The drawing under review shows one solid part. Ordinate dimensions are in mm from its lowest x, y, z. Give positions to 0.01 mm unless a question says otherwise; leave off trailing zeros. Write each loop counter-clockwise with the first axis right and the second up, starting at its lowest first coordinate (ties: lowest second). Pieces come first, ordered by that corner, then holes. Notation, with made-up numbers: M -16.75,18 L 36.25,18 A7 cw 36.25,24 Z; hole C 7,25.25 d10. An arc over 180 degrees is marked long. Answer as a JSON object with one key per item and string values. Group by question number.
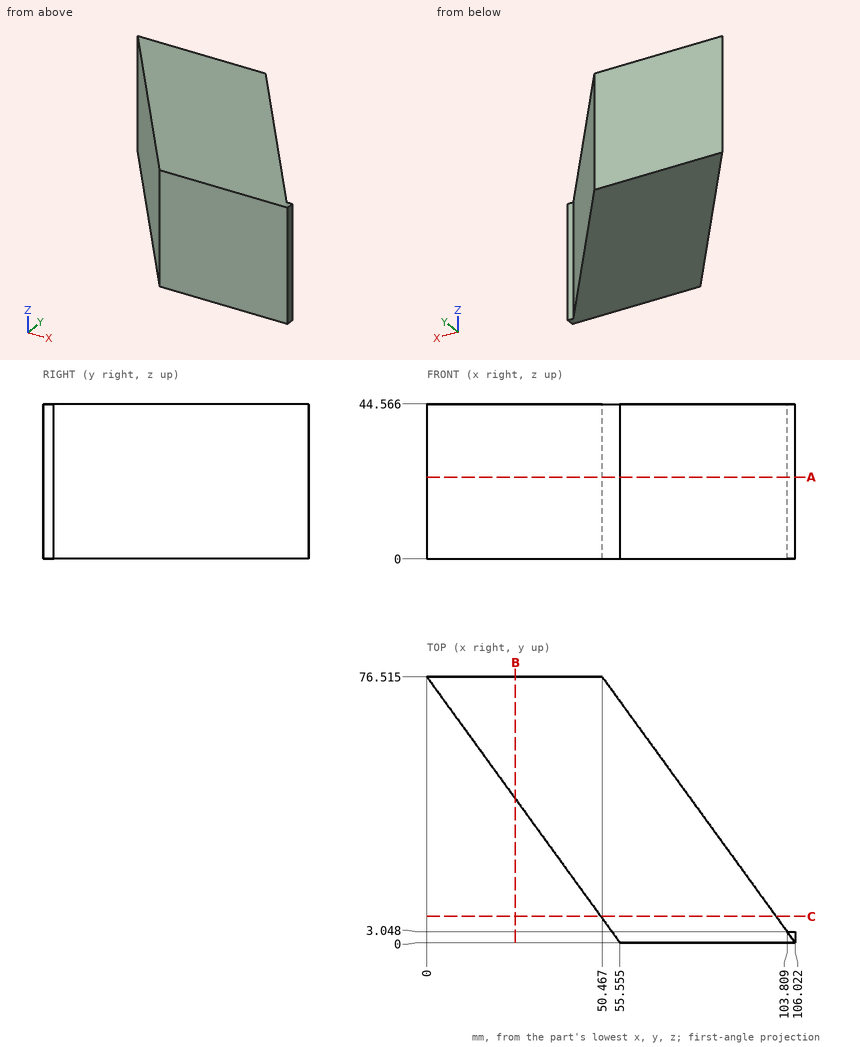
Item 1: To check wall thickness, follow probe 1 along X at (y, z) = (6, 3) (1 decimal); probe 2 along X at (y, z) = (59, 39.5) (1 decimal); probe 3 along Y at (x, z) = (81.5, 6) (1 decimal). State the ranges of each line that lie inside material, in increasing order.
Item 2: Consider section A-A (z = 23.5). Give the boundary of the cut face in (x, y) (1 decimal).
Item 3: Consider section B-B (x = 25.5). Give the boundary of the cut face in (y, z) (1 decimal).
Item 4: Consider section C-C (y = 7.5). Give the boundary of the cut face in (x, z), plus the area to 3 significant figures.
Item 5: Insertion check: P1, Ø3, axis at y = 57.5, z = 25.5, coming from the -X side; P2, Ø6, axis at y = 63, z = 22, coming from the +X side; P3, Ø2.5, axis at x = 105.5, z = 14, coming from the +Y side. Each pin has a flat end and moves straight along its axis. Give the tip position at first contact, or say it passes through.
Result set:
{
 "1": {"probe 1": "x = 51.2 to 101.7", "probe 2": "x = 12.7 to 63.2", "probe 3": "y = 0 to 33.8"},
 "2": {"outline": "M 0,76.5 L 55.6,0 L 106,0 L 106,3 L 103.8,3 L 50.5,76.5 Z"},
 "3": {"outline": "M 41.4,0 L 76.5,0 L 76.5,44.6 L 41.4,44.6 Z"},
 "4": {"outline": "M 50.11,0 L 100.58,0 L 100.58,44.57 L 50.11,44.57 Z", "area": "2,250 mm^2"},
 "5": {"P1": "stops at x = 12.72", "P2": "stops at x = 62.46", "P3": "stops at y = 3.05"}
}
